The model under review builds one solid part; all positions refer to its coordinate system, in mm. Face numbers are marked on the shaded views. A direction names the side the tool comes from. Give positions to 0.01 mm unless a question says otherwise; leave off trailing zeros. Order: outer loops, then holes, each group sorted by start corner. A loop starts at its lowest first (then second) coordinate and runs counter-clockwise, first axis right, second up.
```python
from build123d import *

# Parameters (mm, degrees)
CROQUIS1_R              = 12
CROQUIS1_R_2            = 1.6
CROQUIS1_R_3            = 2.2
SALIENTE_EXTRUIR1_DEPTH = 8


with BuildPart() as part:
    # Croquis1 → Saliente-Extruir1 (new body)
    with BuildSketch(Plane(origin=(0, 0, 0), x_dir=(1, 0, 0), z_dir=(0, 1, 0))):
        Polygon((18, -21), (20.998132752, -18.001867248), (20.998132752, -13.001867248), (23.996265504, -10.003734496), (47.996265504, -10.003734496), (50.994398257, -7.005601743), (50.994398257, 6.994398257), (47.996265504, 9.992531009), (23.996265504, 9.992531009), (20.998132752, 12.990663761), (20.998132752, 17.990663761), (18, 20.988796513), (-18, 20.988796513), (-21.001869571, 17.99439127), (-21.001869571, -18.00560873), (-18, -21), align=None)
        Circle(CROQUIS1_R, mode=Mode.SUBTRACT)
        with Locations((-15.5, -15.5)):
            Circle(CROQUIS1_R_2, mode=Mode.SUBTRACT)
        with Locations((-15.5, 15.5)):
            Circle(CROQUIS1_R_2, mode=Mode.SUBTRACT)
        with Locations((15.5, 15.5)):
            Circle(CROQUIS1_R_2, mode=Mode.SUBTRACT)
        with Locations((15.5, -15.5)):
            Circle(CROQUIS1_R_2, mode=Mode.SUBTRACT)
        with Locations((30.998135075, -0.003734496)):
            Circle(CROQUIS1_R_3, mode=Mode.SUBTRACT)
        with Locations((41.008135075, -0.003734496)):
            Circle(CROQUIS1_R_3, mode=Mode.SUBTRACT)
    extrude(amount=SALIENTE_EXTRUIR1_DEPTH)


solid = part.part
```
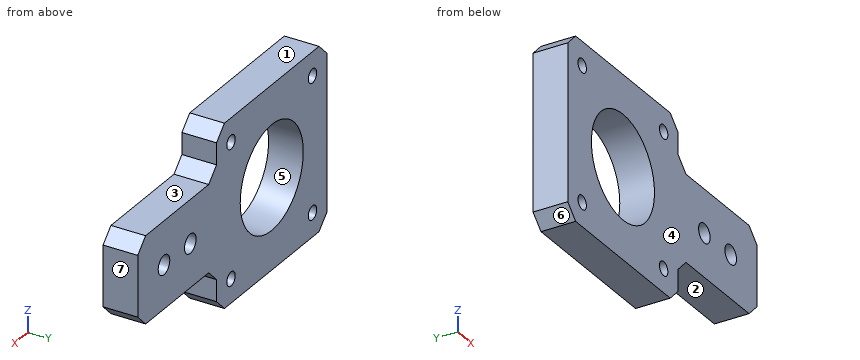
Item 1: Take a section at D-D (y = 6). Give the boundary of the cut face in (x, z), and give its area (3 significant figures).
Values found:
outline: (-21, -17.99) - (-18, -20.99) - (18, -20.99) - (21, -17.99) - (21, -12.99) - (24, -9.99) - (48, -9.99) - (50.99, -6.99) - (50.99, 7.01) - (48, 10) - (24, 10) - (21, 13) - (21, 18) - (18, 21) - (-18, 21) - (-21, 18.01) - close; hole circle Ø3.2 at (-15.5, -15.5); hole circle Ø3.2 at (-15.5, 15.5); hole circle Ø24 at (0, 0); hole circle Ø3.2 at (15.5, -15.5); hole circle Ø3.2 at (15.5, 15.5); hole circle Ø4.4 at (31, 0); hole circle Ø4.4 at (41.01, 0)
area: 1,830 mm2
Item 2: Take a section at C-C (x = 0). Give the boundary of the cut face in (y, z), and give its area (3 significant figures).
Values found:
outline: (0, -20.99) - (8, -20.99) - (8, -12) - (0, -12) - close; (0, 12) - (8, 12) - (8, 21) - (0, 21) - close
area: 144 mm2
Item 3: Take a section at A-A (z = -15.5). Give the boundary of the cut face in (x, y), and give its area (3 significant figures).
Values found:
outline: (-21, 0) - (-17.1, 0) - (-17.1, 8) - (-21, 8) - close; (-13.9, 0) - (13.9, 0) - (13.9, 8) - (-13.9, 8) - close; (17.1, 0) - (21, 0) - (21, 8) - (17.1, 8) - close
area: 285 mm2
Item 4: Take a section at B-B (x = 15.5). Give the boundary of the cut face in (y, z), and give its area (3 significant figures).
Values found:
outline: (0, -20.99) - (8, -20.99) - (8, -17.1) - (0, -17.1) - close; (0, -13.9) - (8, -13.9) - (8, 13.9) - (0, 13.9) - close; (0, 17.1) - (8, 17.1) - (8, 21) - (0, 21) - close
area: 285 mm2
Item 5: Draft analysis for pull direction X (two halves, no side actions). For the marked faces 4, 5, 6 and 7, state which applies: released by +X, released by -X, zero draft, split by the parting line, or undercut.
Values found:
face 4: zero draft
face 5: undercut
face 6: released by -X
face 7: released by +X
Item 6: For line 1 (X direction, y = 5.75, z = 15.5); line 2 (X direction, y = 5, z = 2); line 3 (X direction, y = 5.25, z = -1), list the stretches that pass through material, from the lowest coordinate up.
Values found:
line 1: x = -21 to -17.1, -13.9 to 13.9, 17.1 to 21
line 2: x = -21 to -11.83, 11.83 to 30.07, 31.92 to 40.08, 41.93 to 50.99
line 3: x = -21 to -11.96, 11.96 to 29.04, 32.96 to 39.05, 42.97 to 50.99
Item 7: For the marked faces 1, 2 and 3, list the 3-axis set-ups (+Z, -Z, +X, -X, +Y, -Y) from which the entire face can be reached by the end or side of a thin tool; tool diameter is ignored.
Values found:
face 1: +Z, +X, -X, +Y, -Y
face 2: -Z, +X, +Y, -Y
face 3: +Z, +X, +Y, -Y
Item 8: Clearance check with flat-ended pins moving along their axes: pin 1 Ø2.5 at (x, y) = (35.5, 2) entering from -Z; pin 2 Ø4 at (y, z) = (5.5, -16) entering from +X. State where each tip first meets the part, or that it passes through.
Values found:
pin 1: stops at z = -9.99
pin 2: stops at x = 21
